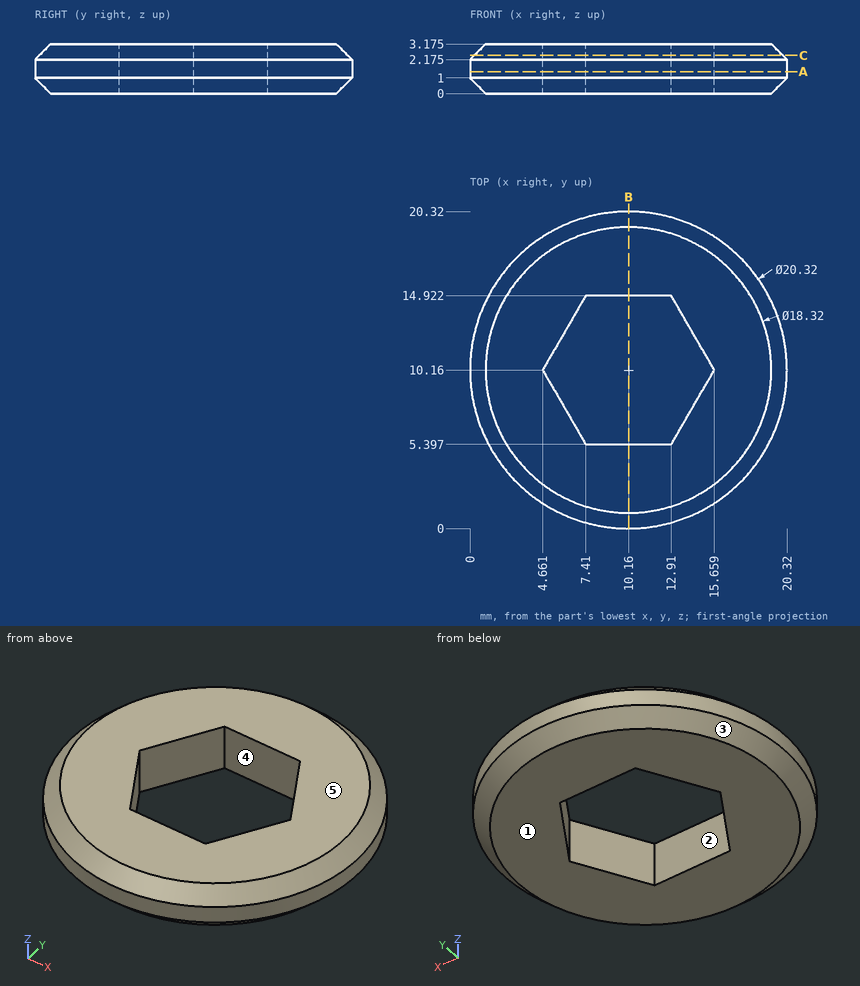
Job drawing, mm, ordinate dimensions from the low corner. One solid piece. A direction names the side the tool comes from. Coordinates: 2 decimals unless noted, no trailing zeros. Write each loop counter-clockwise with the first axis right and the second up, starting at its lowest first coordinate (ties: lowest second). Pieces come first, ordered by that corner, then holes. Notation, with made-up numbers: (18, 7.25) -> (68, 7.25) arc R21 ccw to (68, 13.25) -> close; hole circle Ø2 at (0.5, -38.5). An arc over 180 degrees is marked (long way). Use CSV: the item, a comma, the result in double quotes. Start each with the question number.
Item 1: Two-plate mould, pull along Y, no slides. Class the marked faces 3, 4 and 5: +Y half, -Y half, draft (parallel to the pull), parting line (faces both ways), or undercut.
Item 2: Tool access for the marked faces 1 and 2: list every direction of +Z, -Z, +X, -X, +Y, -Y with a clear straight run to the whole face (end or side of a thin tool).
Item 3: Drop a flat-ended pin along its axis: P1, Ø10, axis at x = 3.5, y = 6.5, coming from the -Z side. Give the stop position or say it passes through.
Item 4: Band-saw the part on B-B, the plane x = 10.16. Write the cut outline in (y, z) (1 decimal).
Item 5: Band-saw the part on A-A, the plane z = 1.4. Write the cut outline in (x, y).
Item 6: Wall check: probe 1 along X at (y, z) = (9, 0.5); probe 2 along Y at (x, z) = (13.25, 0.95) (1 decimal); probe 3 along X at (y, z) = (14.75, 0.8). Give the ranges that are in metal, low to high.
Item 7: Band-saw the part on C-C, the plane z = 2.45. Write the cut outline in (x, y) (1 decimal).
Response values:
1,face 3,"parting line"
1,face 4,"undercut"
1,face 5,"draft"
2,face 1,"-Z, +X, -X, +Y, -Y"
2,face 2,"+Z, -Z"
3,P1,"stops at z = 0"
4,outline,"(0, 1) -> (1, 0) -> (5.4, 0) -> (5.4, 3.2) -> (1, 3.2) -> (0, 2.2) -> close; (14.9, 0) -> (19.3, 0) -> (20.3, 1) -> (20.3, 2.2) -> (19.3, 3.2) -> (14.9, 3.2) -> close"
5,outline,"circle Ø20.32 at (10.16, 10.16); hole (4.66, 10.16) -> (7.41, 5.4) -> (12.91, 5.4) -> (15.66, 10.16) -> (12.91, 14.92) -> (7.41, 14.92) -> close"
6,probe 1,"x = 0.57 to 5.33, 14.99 to 19.75"
6,probe 2,"y = 0.5 to 6, 14.3 to 19.8"
6,probe 3,"x = 1.32 to 7.31, 13.01 to 19"
7,outline,"circle Ø19.8 at (10.2, 10.2); hole (4.7, 10.2) -> (7.4, 5.4) -> (12.9, 5.4) -> (15.7, 10.2) -> (12.9, 14.9) -> (7.4, 14.9) -> close"
